For this review, take the finished solid that the model builds, in its own axes (mm). Round coordinates to 2 decimals unless told otherwise and drop trailing zeros. Order: outer loops, then holes, each group sorted by start corner. A loop starts at its lowest first (then second) coordinate and runs counter-clockwise, first axis right, second up. Notation, with made-up numbers: (-32.5, -14) -> (19.5, -14) arc R25 cw to (19.5, 18) -> close; hole circle Ø2 at (0.5, -31). An arc over 180 degrees is marked (long way). Use a Markdown table: item, result. Add a question column.
1) Consider section A-A (y = -287). State the section outline as (x, z) points, plus the area to 3 significant figures.
2) Consider section D-D (y = -248.5). State the section outline as (x, z) points, plus the area to 3 significant figures.
3) Consider section B-B (x = -145). State the section outline as (y, z) points, plus the area to 4 significant figures.
4) Consider section C-C (x = -82). State the section outline as (y, z) points, plus the area to 3 significant figures.
5) Wall thickness on line 1 along Y through (x, z) = (45.75, 2.1); line 2 along Y through (x, z) = (0.75, 0.95); line 3 along Y through (x, z) = (-22.25, 3.85) (3 decimals): over which ranges is each line inside the solid? List them lowest first. Write a range as [from, to].
6) Clearance check with flat-ended pins moving along their axes: P1, Ø3, axis at x = 25, z = 3.5, coming from the +Y side; P2, Ø3, axis at x = 49.125, y = -91.25, coming from the +Z side; P3, Ø3, axis at x = -162.5, z = 4.5, coming from the -Y side; P4, Ø6, axis at x = -44.25, y = -46.25, coming from the -Z side. State where each tip first meets the part, or that it passes through.
```python
from build123d import *

# Parameters (mm, degrees)
BOSS_EXTRUDE1_DEPTH            = 6.35
FILLET1_R                      = 50
FILLET2_R                      = 30
SKETCH2_R                      = 4.05
CUT_EXTRUDE1_DEPTH             = 390.402519894
SKETCH4_W                      = 19
SKETCH4_H                      = 4
BOSS_EXTRUDE3_DEPTH            = 6.35
CHAMFER1_SIZE                  = 1
CHAMFER1_SIZE2                 = 1.732050808
FILLET3_R                      = 1.5
FILLET8_R                      = 10
CBORE_FOR_M5_SHCS2_D           = 4.75
CBORE_FOR_M5_SHCS2_CBORE_D     = 10
CBORE_FOR_M5_SHCS2_CBORE_DEPTH = 3.1


with BuildPart() as part:
    # Sketch1 → Boss-Extrude1 (new body)
    with BuildSketch(Plane.XY):
        Polygon((53.625, -52.25), (53.625, -40.25), (40.25, -40.25), (-40.25, -40.25), (-53.625, -40.25), (-53.625, -52.25), align=None)
        with BuildLine():
            Line((53.625, -140.25), (53.625, -52.25))
            Line((53.625, -52.25), (-53.625, -52.25))
            Line((-53.625, -52.25), (-187.067700458, -259.975777937))
            ThreePointArc((-187.067700458, -259.975777937), (-175.291577032, -326.779647572), (-107.761575635, -320.366146777))
            Line((-107.761575635, -320.366146777), (53.625, -140.25))
        make_face()
    extrude(amount=BOSS_EXTRUDE1_DEPTH)

    # Fillet1
    fillet1_edges = [part.edges().sort_by_distance(p)[0] for p in [
        (53.625, -140.25, 3.175),
    ]]
    fillet(fillet1_edges, radius=FILLET1_R)

    # Fillet2
    fillet2_edges = [part.edges().sort_by_distance(p)[0] for p in [
        (-53.625, -52.25, 3.175),
    ]]
    fillet(fillet2_edges, radius=FILLET2_R)

    # Sketch2 → Cut-Extrude1 (cut, through all)
    with BuildSketch(Plane(origin=(0, 0, 0), x_dir=(-1, 0, 0), z_dir=(0, 0, -1))):
        with Locations((145, -287)):
            Circle(SKETCH2_R)
    extrude(amount=-CUT_EXTRUDE1_DEPTH, mode=Mode.SUBTRACT)

    # Sketch4 → Boss-Extrude3 (add)
    with BuildSketch(Plane(origin=(0, 0, 0), x_dir=(-1, 0, 0), z_dir=(0, 0, -1))):
        with Locations((2.875, -38.25)):
            Rectangle(SKETCH4_W, SKETCH4_H)
    extrude(amount=-BOSS_EXTRUDE3_DEPTH)

    # Chamfer1
    chamfer1_edges = [part.edges().sort_by_distance(p)[0] for p in [
        (-12.375, -36.25, 3.175),
        (6.625, -36.25, 3.175),
    ]]
    chamfer1_side = [part.faces().sort_by_distance(p)[0] for p in [
        (-2.875, -36.25, 3.175),
    ]]
    chamfer(chamfer1_edges, length=CHAMFER1_SIZE, length2=CHAMFER1_SIZE2, reference=chamfer1_side[0])

    # Fillet3
    fillet3_edges = [part.edges().sort_by_distance(p)[0] for p in [
        (-12.375, -40.25, 3.175),
        (6.625, -40.25, 3.175),
    ]]
    fillet(fillet3_edges, radius=FILLET3_R)

    # Fillet8
    # the kernel refuses this fillet: 10 mm, written as the material it takes off along each edge
    with BuildSketch(Plane(origin=(53.625, -40.25, -25), x_dir=(-1, 0, 0), z_dir=(0, 0, 1))) as fillet8_piece_1:
        with BuildLine():
            CenterArc((FILLET8_R, FILLET8_R), FILLET8_R, 180, 90)
            Line((0, FILLET8_R), (0, 0))
            Line((0, 0), (FILLET8_R, 0))
        make_face()
    extrude(amount=56.35, mode=Mode.SUBTRACT)
    with BuildSketch(Plane(origin=(-53.625, -40.25, -23.541918235), x_dir=(1, 0, 0), z_dir=(0, 0, 1))) as fillet8_piece_2:
        with BuildLine():
            CenterArc((9.416767294, -10), FILLET8_R, 90, 80.203799094)
            Line((-0.43742453, -8.298558404), (-1.422843712, -8.128414244))
            ThreePointArc((-1.422843712, -8.128414244), (-1, -3.194233614), (-1, 0))
            Line((-1, 0), (0, 1))
            Line((0, 1), (9.416767294, 1))
            Line((9.416767294, 1), (9.416767294, 0))
        make_face()
    extrude(amount=53.43383647, mode=Mode.SUBTRACT)

    # CBORE for M5 SHCS2 (through all)
    with Locations(Plane(origin=(0, 0, 0), x_dir=(-1, 0, 0), z_dir=(0, 0, -1))):
        with Locations((-45.75, 26.75), (-45.75, -46.25), (-23.75, -54.25), (-0.75, -46.25), (22.25, -54.25), (44.25, -46.25), (-49.125, -91.25)):
            CounterBoreHole(CBORE_FOR_M5_SHCS2_D / 2, CBORE_FOR_M5_SHCS2_CBORE_D / 2, CBORE_FOR_M5_SHCS2_CBORE_DEPTH)


solid = part.part
```
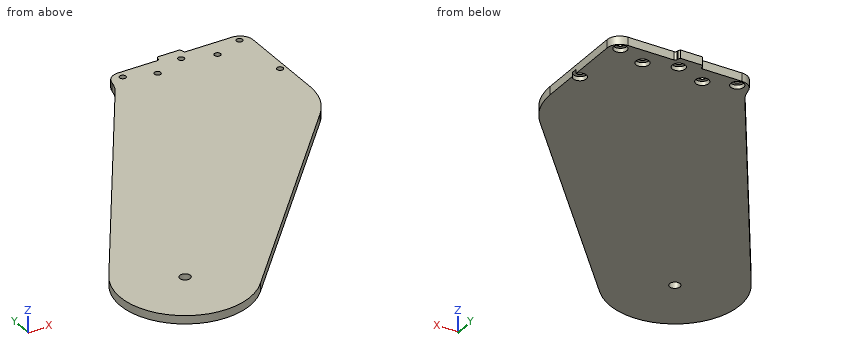
Results list:
| question | item | result |
|---|---|---|
| 1 | outline | (-195, 0) -> (-149.05, 0) -> (-149.05, 6.35) -> (-195, 6.35) -> close; (-140.95, 0) -> (-77.87, 0) -> (-77.87, 6.35) -> (-140.95, 6.35) -> close |
| 1 | area | 692 mm2 |
| 2 | outline | (-179.7, 0) -> (-43.37, 0) -> (-43.37, 6.35) -> (-179.7, 6.35) -> close |
| 2 | area | 866 mm2 |
| 3 | outline | (-337, 0) -> (-291.05, 0) -> (-291.05, 6.35) -> (-337, 6.35) -> close; (-282.95, 0) -> (-194.49, 0) -> (-194.49, 6.35) -> (-282.95, 6.35) -> close |
| 3 | area | 853.5 mm2 |
| 4 | outline | (-291.61, 0) -> (-96.42, 0) -> (-96.42, 6.35) -> (-291.61, 6.35) -> close |
| 4 | area | 1,240 mm2 |
| 5 | line 1 | [-148.06, -94.94], [-87.56, -51.25], [-41.25, -40.48] |
| 5 | line 2 | [-199.26, -51.25], [-41.25, -36.25] |
| 5 | line 3 | [-224.931, -56.625], [-51.875, -40.25] |
| 6 | P1 | y = -40.25 |
| 6 | P2 | through |
| 6 | P3 | y = -334.37 |
| 6 | P4 | z = 3.1 |
